Autodesk Inventor part; units mm, degrees
ref_plane "YZ Plane" through (0, 0, 0) normal (1, 0, 0) x (0, 1, 0)
ref_plane "XZ Plane" through (0, 0, 0) normal (0, 1, 0) x (-1, 0, 0)
ref_plane "XY Plane" through (0, 0, 0) normal (0, 0, 1) x (1, 0, 0)
sketch "스케치2" plane through (0, 0, 0) normal (0, 1, 0) x (-1, 0, 0)
  line L0 (15, 15) -> (-15, 15)
  line L1 (-15, 15) -> (-15, -15)
  line L2 (-15, -15) -> (15, -15)
  line L3 (15, -15) -> (15, 15)
  line L4 (15, 15) -> (-15, -15) construction
  line L5 (-15, 15) -> (15, -15) construction
  circle A0 centre (15, -15) radius 2.6
  circle A1 centre (-15, -15) radius 2.6
  circle A2 centre (15, 15) radius 2.6
  circle A3 centre (-15, 15) radius 2.6
  line L6 (21, -21) -> (-21, -21)
  line L7 (-21, -21) -> (-21, 21)
  line L8 (-21, 21) -> (21, 21)
  line L9 (21, 21) -> (21, -21)
  line L10 (10.05, 10.05) -> (-10.05, 10.05)
  line L11 (-10.05, 10.05) -> (-10.05, -10.05)
  line L12 (-10.05, -10.05) -> (10.05, -10.05)
  line L13 (10.05, -10.05) -> (10.05, 10.05)
  line L14 (10.05, 10.05) -> (-10.05, -10.05) construction
  line L15 (-10.05, 10.05) -> (10.05, -10.05) construction
  line L16 (-15.05, -15.05) -> (-15.05, 15.05)
  line L17 (-15.05, 15.05) -> (15.05, 15.05)
  line L18 (15.05, 15.05) -> (15.05, -15.05)
  line L19 (15.05, -15.05) -> (-15.05, -15.05)
  point P0 (0, 0)
  dimension "d16" = 30
  dimension "d17" = 30
  dimension "d18" = 5.2
  dimension "d21" = 30
  dimension "d24" = 30
  dimension "d27" = 6
  dimension "d28" = 20.1
  dimension "d29" = 20.1
  dimension "d30" = 5
extrude "돌출2" add sketch "스케치2" along normal blind 5 contours A3 L17 A2 L0 | L0 A2 L3 A0 L2 A1 L1 A3 | L1 A1 L16 A3 | A2 L18 A0 L3 | L2 A0 L19 A1 | L6 L7 L8 L9 | L13 L12 L11 L10
sketch "스케치3" plane through (0, 5, 0) normal (0, 1, 0) x (1, 0, 0)
  line L0 (-10.05, 10.05) -> (10.05, 10.05)
  line L1 (10.05, 10.05) -> (10.05, -10.05)
  line L2 (10.05, -10.05) -> (-10.05, -10.05)
  line L3 (-10.05, -10.05) -> (-10.05, 10.05)
  line L4 (-10.05, 10.05) -> (10.05, -10.05) construction
  line L5 (10.05, 10.05) -> (-10.05, -10.05) construction
  line L6 (13.05, 13.05) -> (-13.05, 13.05)
  line L7 (-13.05, 13.05) -> (-13.05, -13.05)
  line L8 (-13.05, -13.05) -> (13.05, -13.05)
  line L9 (13.05, -13.05) -> (13.05, 13.05)
  point P0 (0, 0)
  dimension "d33" = 20.1
  dimension "d34" = 20.1
  dimension "d35" = 3
extrude "돌출3" add sketch "스케치3" along normal blind 60
fillet "모깎기1" radius 3 12 edges at (-21, 5, 0) (0, 5, -21) (0, 5, 21) (21, 5, 0) (-21, 2.5, -21) (-21, 2.5, 21) (21, 2.5, 21) (21, 2.5, -21) (-13.05, 35, 13.05) (13.05, 35, 13.05) (13.05, 35, -13.05) (-13.05, 35, -13.05)
properties part number "Profile_Plate_Holder"
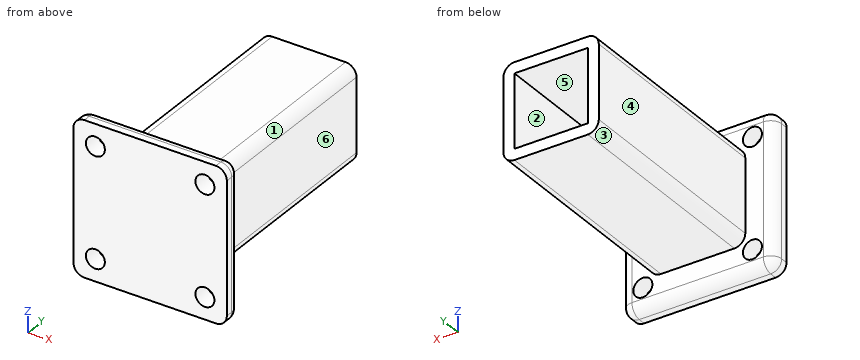
Geometry check sheet. Reference: the model listing, model coordinates, mm. Face numbers are marked on the shaded views. A direction names the side the tool comes from. Coordinates: 2 decimals unless noted, no trailing zeros. Order: outer loops, then holes, each group sorted by start corner. A loop starts at its lowest first (then second) coordinate and runs counter-clockwise, first axis right, second up. Notation, with made-up numbers: (-21, 84) - (38, 84) arc R11 cw to (38, 102) - close; hole circle Ø6 at (5, 37). An arc over 180 degrees is marked (long way). Use one line per item in the form item = value.
1. Section check B-B (y = 18). Record the boundary of the cut face in (x, z).
Here are the results:
outline = (-13.05, -10.05) arc R3 ccw to (-10.05, -13.05) - (10.05, -13.05) arc R3 ccw to (13.05, -10.05) - (13.05, 10.05) arc R3 ccw to (10.05, 13.05) - (-10.05, 13.05) arc R3 ccw to (-13.05, 10.05) - close; hole (-10.05, -10.05) - (10.05, -10.05) - (10.05, 10.05) - (-10.05, 10.05) - close
2. Section check C-C (x = -15). Record the boundary of the cut face in (y, z), then the cut area to 3 significant figures.
Here are the results:
outline = (0, -21) - (2, -21) arc R3 ccw to (5, -18) - (5, -17.6) - (0, -17.6) - close; (0, -12.4) - (5, -12.4) - (5, 12.4) - (0, 12.4) - close; (0, 17.6) - (5, 17.6) - (5, 18) arc R3 ccw to (2, 21) - (0, 21) - close
area = 154 mm²
3. Section check D-D (z = 6). Record the boundary of the cut face in (x, y), then the cut area to 3 significant figures.
Here are the results:
outline = (-21, 0) - (21, 0) - (21, 2) arc R3 ccw to (18, 5) - (13.05, 5) - (13.05, 65) - (10.05, 65) - (10.05, 5) - (-10.05, 5) - (-10.05, 65) - (-13.05, 65) - (-13.05, 5) - (-18, 5) arc R3 ccw to (-21, 2) - close
area = 566 mm²
4. Gauge pin test, flat ends, axial feed: pin 1 (1 mm diameter, centred on y = 8, z = -8, fed in from +X); pin 2 (5 mm diameter, centred on x = 14, y = 27.5, fed in from +Z); pin 3 (3 mm diameter, centred on x = -6, y = 26, fed in from +Z); pin 4 (8.5 mm diameter, centred on x = -15, z = 15, fed in from +Y). Record the tip position at first contact, or that the pin passes through.
Here are the results:
pin_1 = 13.05
pin_2 = 12.68
pin_3 = 13.05
pin_4 = 65
5. Section check A-A (z = 15). Record the boundary of the cut face in (x, y).
Here are the results:
outline = (-21, 0) - (-17.6, 0) - (-17.6, 5) - (-18, 5) arc R3 ccw to (-21, 2) - close; (-12.4, 0) - (12.4, 0) - (12.4, 5) - (-12.4, 5) - close; (17.6, 0) - (21, 0) - (21, 2) arc R3 ccw to (18, 5) - (17.6, 5) - close
6. Access from +Z, -Z, +X, -X, +Y, -Y to the whole of each face (thin tool, end or side, straight path). Record for the marked faces 4, 5 and 6.
Here are the results:
face_4 = +Z, -Z, -X, +Y
face_5 = +Y
face_6 = +Z, -Z, +X, +Y
7. Scan lines: line 1 (X direction, y = 1.1, z = 15); line 2 (Z direction, x = -15, y = 2.25); line 3 (Z direction, x = 3.5, y = 12.5). Record each from-to range of solid material in increasing order.
Here are the results:
line_1 = -21 to -17.6, -12.4 to 12.4, 17.6 to 21
line_2 = -20.99 to -17.6, -12.4 to 12.4, 17.6 to 20.99
line_3 = -13.05 to -10.05, 10.05 to 13.05
8. Draft check along X on the marked faces 1, 2 and 3. Enter one of: pulls with the +X half, pulls with the -X half, needs draft (parallel to the pull), parting line crosses it, or undercut.
Here are the results:
face_1 = pulls with the +X half
face_2 = undercut
face_3 = pulls with the -X half
